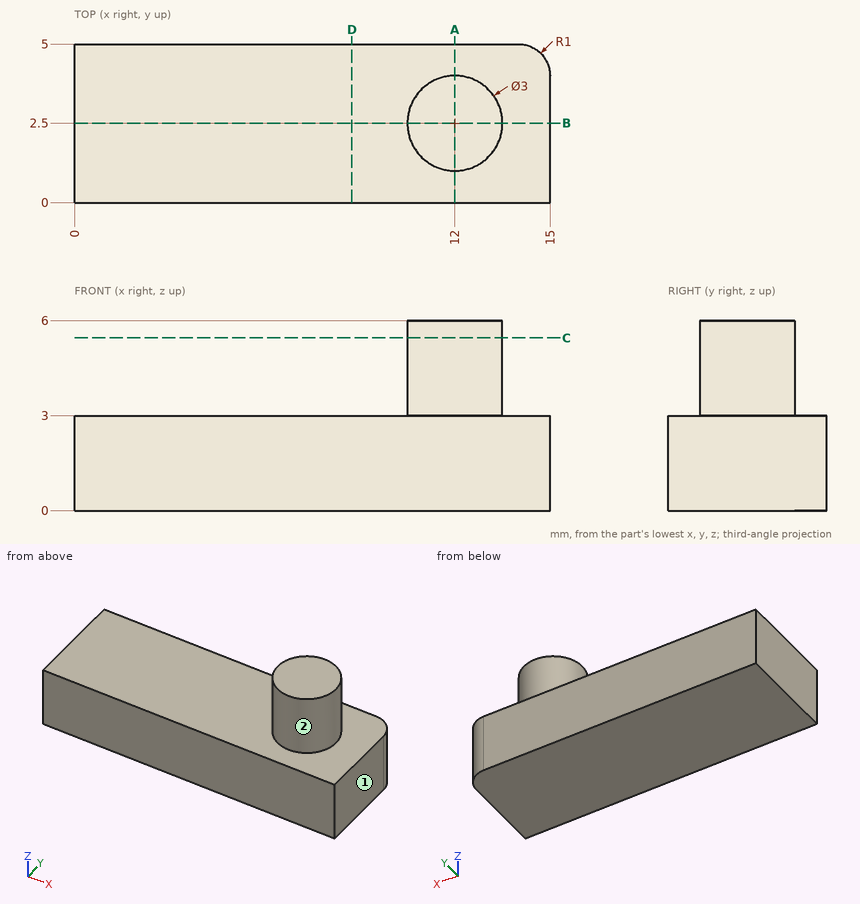
The drawing under review shows one solid part. Ordinate dimensions are in mm from its lowest x, y, z. A direction names the side the tool comes from. Round coordinates to 2 decimals unless told otherwise and drop trailing zeros. Order: outer loops, then holes, each group sorted by start corner. A loop starts at its lowest first (then second) coordinate and runs counter-clockwise, first axis right, second up. Notation, with made-up numbers: (0, -1) -> (14, -1) arc R26 ccw to (14, 23) -> close; hole circle Ø11 at (30.25, 75). An arc over 180 degrees is marked (long way). Return JSON: item names as keys, results as strings.
1. Take a section at B-B (y = 2.5). Write out the cut boundary in (x, z), then the cut area to 3 significant figures.
Answer block:
{"outline": "(0, 0) -> (15, 0) -> (15, 3) -> (13.5, 3) -> (13.5, 6) -> (10.5, 6) -> (10.5, 3) -> (0, 3) -> close", "area": "54.0 mm²"}
2. For L1, parallel to Z at x = 5, y = 2.9; L2, parallel to X at y = 4.85, z = 0.65; L3, parallel to X at y = 3.75, z = 3.6, list the stretches that pass through material, from the lowest coordinate up. Write a range as [from, to].
Answer block:
{"L1": "z = [0, 3]", "L2": "x = [0, 14.53]", "L3": "x = [11.17, 12.83]"}
3. Take a section at D-D (x = 8.75). Write out the cut boundary in (y, z), then the cut area to 3 significant figures.
Answer block:
{"outline": "(0, 0) -> (5, 0) -> (5, 3) -> (0, 3) -> close", "area": "15.0 mm²"}
4. Take a section at A-A (x = 12). Write out the cut boundary in (y, z), then the cut area to 3 significant figures.
Answer block:
{"outline": "(0, 0) -> (5, 0) -> (5, 3) -> (4, 3) -> (4, 6) -> (1, 6) -> (1, 3) -> (0, 3) -> close", "area": "24.0 mm²"}
5. Take a section at C-C (z = 5.45). Write out the cut boundary in (x, y).
Answer block:
{"outline": "circle Ø3 at (12, 2.5)"}
6. For the marked faces 1 and 2, list the 3-axis set-ups (+Z, -Z, +X, -X, +Y, -Y) from which the entire face can be reached by the end or side of a thin tool; tool diameter is ignored.
Answer block:
{"face 1": "+Z, -Z, +X, +Y, -Y", "face 2": "+Z"}
